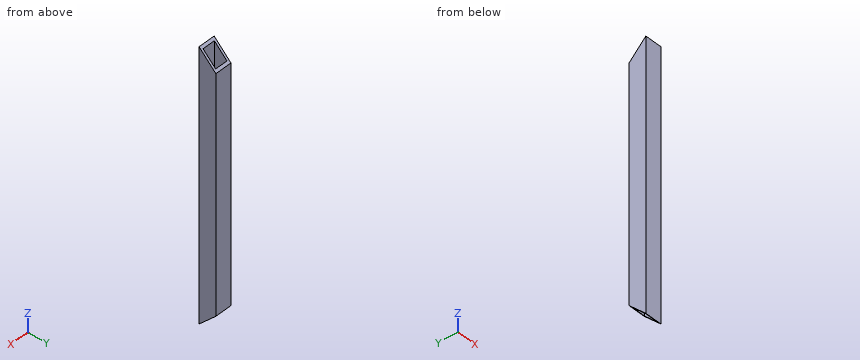
from build123d import *

# Parameters (mm, degrees)
F0_W     = 38.1
F0_H     = 38.1
F0_W_2   = 28.5496
F0_H_2   = 28.5496
F1_DEPTH = 609.6
F3_DEPTH = 38.101
F4_DEPTH = 38.101


with BuildPart() as f1:
    # F0 (on Top) → F1 (new body)
    with BuildSketch(Plane.XY):
        Rectangle(F0_W, F0_H)
        Rectangle(F0_W_2, F0_H_2, mode=Mode.SUBTRACT)
    extrude(amount=F1_DEPTH)

    # F2 (on face) → F3 (cut, through all)
    with BuildSketch(Plane.YZ.offset(19.05)):
        Polygon((19.05, 38.1), (-19.05, 0), (19.05, 0), align=None)
    extrude(amount=-F3_DEPTH, mode=Mode.SUBTRACT)

    # F2 (on face) → F4 (cut, through all)
    with BuildSketch(Plane.YZ.offset(19.05)):
        Polygon((19.05, 609.6), (-19.05, 609.6), (19.05, 571.5), align=None)
    extrude(amount=-F4_DEPTH, mode=Mode.SUBTRACT)


solid = f1.part
Input: part model. Units: mm. Frame: model coordinates. Coordinates: 2 decimals unless noted, no trailing zeros. Order: outer loops, then holes, each group sorted by start corner. A loop starts at its lowest first (then second) coordinate and runs counter-clockwise, first axis right, second up. Notation, with made-up numbers: M 63,19.25 L 89,19.25 A23 ccw 89,50.25 Z; hole C 63,-34 d8. An arc over 180 degrees is marked long. One line per question, with ' | ' between items.
Item 1: Section A-A (y = -8). Output: boundary loops of the cut face in (x, z).
Geometry results:
outline: M -19.05,11.05 L -14.27,11.05 L -14.27,598.55 L -19.05,598.55 Z; M 14.27,11.05 L 19.05,11.05 L 19.05,598.55 L 14.27,598.55 Z
Item 2: Section C-C (x = 9). Output: boundary loops of the cut face in (y, z).
Geometry results:
outline: M -19.05,0 L -14.27,4.78 L -14.27,604.82 L -19.05,609.6 Z; M 14.27,33.32 L 19.05,38.1 L 19.05,571.5 L 14.27,576.28 Z
Item 3: Pin query (flat end, axial travel): pin 1 (8 mm diameter, centred on x = 11.5, y = -14.5, fed in from -Z); pin 2 (1.5 mm diameter, centred on x = 8, y = 14, fed in from -Z); pin 3 (10 mm diameter, centred on x = -10.5, y = 6, fed in from -Z). Return the tip coordinate at first contact, or that it passes through.
Geometry results:
pin 1: stops at z = 0.55 | pin 2: stops at z = 33.32 | pin 3: stops at z = 21.77
Item 4: Ray query, line 1 along Y through (x, z) = (-13, 284); line 2 along Z through (x, y) = (-15, 8). Return the intervals inside material, ascending.
Geometry results:
line 1: y = -19.05 to -14.27, 14.27 to 19.05 | line 2: z = 27.05 to 582.55
Item 5: Section B-B (z = 155). Output: boundary loops of the cut face in (x, y).
Geometry results:
outline: M -19.05,-19.05 L 19.05,-19.05 L 19.05,19.05 L -19.05,19.05 Z; hole M -14.27,-14.27 L 14.27,-14.27 L 14.27,14.27 L -14.27,14.27 Z
